Read the model definition and answer for the solid it produces. Units are mm, in the model's axes. A direction names the side the tool comes from. Coordinates: 2 decimals unless noted, no trailing zeros. Loops run counter-clockwise (first coordinate to the right, second up) from the corner with the lowest first, then second, coordinate; pieces in that order, holes last. Notation, with made-up numbers: M -35.75,72.5 L 13.25,72.5 A15 cw 13.25,78.5 Z; hole C -31,22.5 d6. An arc over 180 degrees is marked long. One line per item, written item: value. Start each with the question number.
```python
from build123d import *

# Parameters (mm, degrees)
SKETCH1_R           = 95.25
BOSS_EXTRUDE1_DEPTH = 48.26
SKETCH2_R           = 88.9
CUT_EXTRUDE1_DEPTH  = 45.72
SKETCH3_R           = 3.875
BOSS_EXTRUDE4_DEPTH = 11
CIRPATTERN1_COUNT   = 3
SKETCH8_W           = 48.096
SKETCH8_H           = 48.096
SKETCH8_W_2         = 43.016
SKETCH8_H_2         = 43.016
BOSS_EXTRUDE5_DEPTH = 7.62
SKETCH10_W          = 38.096
SKETCH10_H          = 7.62
CUT_EXTRUDE2_DEPTH  = 2.54


with BuildPart() as part:
    # Sketch1 → Boss-Extrude1 (new body)
    with BuildSketch(Plane(origin=(0, 0, 0), x_dir=(1, 0, 0), z_dir=(0, 1, 0))):
        with Locations(Location((0, 0, 0), (0, 0, 90))):
            Circle(SKETCH1_R)
    extrude(amount=BOSS_EXTRUDE1_DEPTH)

    # Sketch2 → Cut-Extrude1 (cut)
    with BuildSketch(Plane(origin=(0, 48.26, 0), x_dir=(1, 0, 0), z_dir=(0, 1, 0))):
        with Locations(Location((0, 0, 0), (0, 0, 270))):
            Circle(SKETCH2_R)
    extrude(amount=-CUT_EXTRUDE1_DEPTH, mode=Mode.SUBTRACT)

    # Sketch3 → Boss-Extrude4 (add)
    with BuildSketch(Plane(origin=(0, 0, 88.9), x_dir=(-1, 0, 0), z_dir=(0, 0, -1))):
        with Locations((1.626800498, 39.26)):
            Circle(SKETCH3_R)
    boss_extrude4 = extrude(amount=BOSS_EXTRUDE4_DEPTH)

    # CirPattern1: Boss-Extrude4 ×3 about axis
    cirpattern1_axis = Axis((0, 0, 0), (0, 1, 0))
    for i in range(1, CIRPATTERN1_COUNT):
        add(boss_extrude4.rotate(cirpattern1_axis, i * 360 / CIRPATTERN1_COUNT))

    # Sketch8 → Boss-Extrude5 (add)
    with BuildSketch(Plane(origin=(0, 2.54, 0), x_dir=(1, 0, 0), z_dir=(0, 1, 0))):
        with Locations((-6.666911053, -54.455125388)):
            Rectangle(SKETCH8_W, SKETCH8_H)
        with Locations((-6.666911053, -54.455125388)):
            Rectangle(SKETCH8_W_2, SKETCH8_H_2, mode=Mode.SUBTRACT)
    extrude(amount=BOSS_EXTRUDE5_DEPTH)

    # Sketch10 → Cut-Extrude2 (cut)
    with BuildSketch(Plane(origin=(0, 0, 30.407125388), x_dir=(-1, 0, 0), z_dir=(0, 0, -1))):
        with Locations((6.666911053, 6.35)):
            Rectangle(SKETCH10_W, SKETCH10_H)
    extrude(amount=-CUT_EXTRUDE2_DEPTH, mode=Mode.SUBTRACT)


solid = part.part
```
1) Section B-B (z = 0) is taken. Determine the outline of the cut face in (x, y).
2) Section D-D (x = 10) is taken. Determine the outline of the cut face in (y, z), then the cut area to 3 significant figures.
3) Consider line 1 along X through (y, z) = (12.5, 0); line 2 along Y through (x, z) = (-3, -57); line 3 along X through (y, z) = (30.5, 22). Determine where each line is inside the solid, lowest interval first.
4) Flat-ended cylindrical pins translate along their axes: pin 1 (6 mm diameter, centred on x = -31, y = 24.5, fed in from -Z); pin 2 (4 mm diameter, centred on x = -7.5, y = 6, fed in from +Z); pin 3 (1.5 mm diameter, centred on x = -52, z = 40.5, fed in from +Y); pin 4 (4 mm diameter, centred on x = -1.5, y = 39, fed in from -Z). Find the tip coordinate at first contact, or state that the pin passes through.
5) Section C-C (y = 39.26) is taken. Determine the outline of the cut face in (x, z), then the cut area to 3 significant figures.
6) A tool of negligible diameter and unlimited length cuts with its end or side. For faces 5 (the face through (-1, 0, 1)), 6 (the face through (17.381, 6, 55)), from which of +Z, -Z, +X, -X, +Y, -Y can it reach the whole face along a straight path? Write none if from no direction.
7) Section A-A (y = 6) is taken. Determine the outline of the cut face in (x, z), then the cut area to 3 significant figures.
8) For a pull along Z with two mould halves and no side action, classify faces 1 (the face through (74.96, 25.72, 47.79)), 2 (the face through (-43, 48.26, 78)), 3 (the face through (92.985, 23.792, 20.648)), 4 (the face through (68.25, 39.31, -37.59)) as released by +Z, released by -Z, zero draft, split by the parting line, or undercut.
Results found:
1. outline: M -95.25,0 L 95.25,0 L 95.25,48.26 L 88.9,48.26 L 88.9,2.54 L -88.9,2.54 L -88.9,48.26 L -95.25,48.26 Z
2. outline: M 0,-94.72 L 48.26,-94.72 L 48.26,-88.34 L 2.54,-88.34 L 2.54,75.96 L 10.16,75.96 L 10.16,78.5 L 2.54,78.5 L 2.54,88.34 L 48.26,88.34 L 48.26,94.72 L 0,94.72 Z
2. area: 1,080 mm²
3. line 1: x = -95.25 to -88.9, 88.9 to 95.25
3. line 2: y = 0 to 2.54
3. line 3: x = -92.67 to -86.13, 86.13 to 92.67
4. pin 1: stops at z = -91.04
4. pin 2: stops at z = 95.09
4. pin 3: stops at y = 2.54
4. pin 4: stops at z = -95.25
5. outline: C 0,0 d190.5; hole M -78.09,-42.49 L -68.59,-37 L -64.71,-43.71 L -74.09,-49.13 A88.9 ccw 75.84,-46.38 L 66.34,-40.9 L 70.21,-34.19 L 79.59,-39.6 A88.9 ccw 2.25,88.87 L 2.25,77.9 L -5.5,77.9 L -5.5,88.73 A88.9 ccw Z
5. area: 3,930 mm²
6. face 5: +Z, -Z, +X, -X, -Y
6. face 6: +Y
7. outline: C 0,0 d190.5; M -30.71,30.41 L -25.71,30.41 L -25.71,32.95 L -28.17,32.95 L -28.17,75.96 L 14.84,75.96 L 14.84,32.95 L 12.38,32.95 L 12.38,30.41 L 17.38,30.41 L 17.38,78.5 L -30.71,78.5 Z; hole C 0,0 d177.8
7. area: 4,040 mm²
8. face 1: undercut
8. face 2: zero draft
8. face 3: split by the parting line
8. face 4: undercut
